Can you work these out from the model? Positions are in its coordinate system, mm. Face numbers are marked on the shaded views. A direction names the side the tool comes from. Round coordinates to 2 decimals unless told otherwise and drop trailing zeros. Loops run counter-clockwise (first coordinate to the right, second up) from the corner with the lowest first, then second, coordinate; pieces in that order, holes last.
(1) Which directions (+Z, -Z, +X, -X, +Y, -Y) give clear straight access to the entire face, cutting with the end or side of a thin tool? Please do the marked faces 5, 6 and 7.
(2) Will these pins go through, and if not, where does the flat tip stop? pin 1 Ø9 at (x, y) = (-27.5, 355) entering from +Z; pin 2 Ø14.5 at (x, y) = (-257.5, 35) entering from +Z; pin 3 Ø3 at (x, y) = (-41.5, 179) entering from -Z; pin 4 Ø21.5 at (x, y) = (-267.5, 30) entering from +Z.
(3) I want a section at B-B on x = -94.5. Write out the boundary of the cut face in (y, z), plus the area to 3 significant figures.
(4) If I drill on line 1 along Y through (x, z) = (-17, 10); line 2 along X through (y, z) = (195, 36); line 3 along X through (y, z) = (349, 14.25), over which ranges is the centre line in solid material (lowest first)?
(5) Thinking about a two-plate mould opening in Y: for the marked faces 1, 2, 3 and 4, which applies, released by +Y, released by -Y, zero draft, split by the parting line, or undercut?
(6) I want a section at A-A on y = 195. Write out the boundary of the cut face in (x, z), plus the area to 3 significant figures.
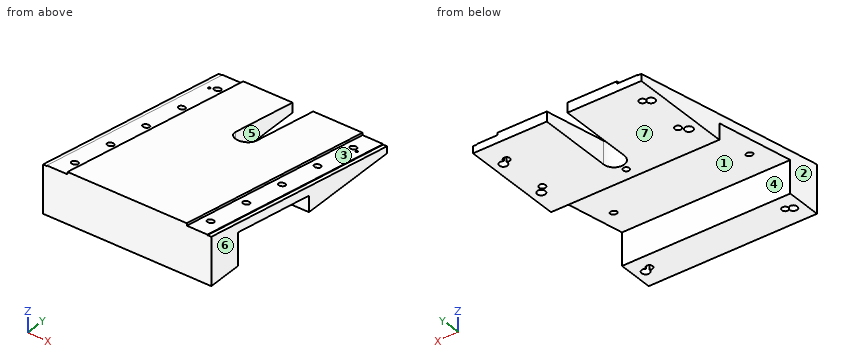
from build123d import *

# Parameters (mm, degrees)
F1_DEPTH  = 285
F3_DEPTH  = 41.5
F5_DEPTH  = 6.5
F7_DEPTH  = 41.5
F8_DEPTH  = 6.5
F13_D     = 11
F15_D     = 13.5
F15_DEPTH = 18
F15_START = 0.4782643
F15_TIP   = 4.0558091784
F17_DEPTH = 85.6227357069
F19_D     = 10
F19_DEPTH = 12
F19_TIP   = 3.0043030951


# Not quite as in the source:
# - a feature names something its author has since deleted; it is built from what else it names


with BuildPart() as f1:
    # F0 (on Right) → F1 (new body)
    with BuildSketch(Plane.YZ):
        Polygon((60, 55.2), (0, 65.8), (0, 0), (60, 0), align=None)
        Polygon((394, 17.0782642931), (0, 86.1), (0, 65.8), (60, 55.2), (219, 27.6782642931), (219, 0.4782642931), (394, 0.4782642931), align=None)
    extrude(amount=-F1_DEPTH)

    # F2 (on face) → F3 (cut)
    with BuildSketch(Plane.YZ):
        Polygon((394, 17.0782642931), (0, 86.1), (0, 82.1), (394, 13.0782642931), align=None)
    extrude(amount=-F3_DEPTH, mode=Mode.SUBTRACT)

    # F4 (on face) → F5 (cut)
    with BuildSketch(Plane.YZ):
        Polygon((394, 13.0782642931), (0, 82.1), (0, 81.1), (394, 12.0782642931), align=None)
    extrude(amount=-F5_DEPTH, mode=Mode.SUBTRACT)

    # F6 (on face) → F7 (cut)
    with BuildSketch(Plane(origin=(-285, 0, 0), x_dir=(0, -1, 0), z_dir=(-1, 0, 0))):
        Polygon((0, 86.1), (-394, 17.0782642931), (-394, 13.0782642931), (0, 82.1), align=None)
    extrude(amount=-F7_DEPTH, mode=Mode.SUBTRACT)

    # F6 (on face) → F8 (cut)
    with BuildSketch(Plane(origin=(-285, 0, 0), x_dir=(0, -1, 0), z_dir=(-1, 0, 0))):
        Polygon((0, 82.1), (-394, 13.0782642931), (-394, 12.0782642931), (0, 81.1), align=None)
    extrude(amount=-F8_DEPTH, mode=Mode.SUBTRACT)

    # F13 (through all)
    with Locations(Plane.XY.offset(86.1)):
        with Locations((-257.5, 355), (-257.5, 275), (-257.5, 195), (-27.5, 355), (-27.5, 275), (-27.5, 195), (-27.5, 115), (-27.5, 35), (-257.5, 115), (-257.5, 35)):
            Hole(F13_D / 2)

    # F15
    # its depths count from where the whole tool has entered the part; down to there all is cleared
    with Locations(Plane(origin=(0, 0, 0), x_dir=(1, 0, 0), z_dir=(0, 0, -1))):
        with Locations((-17.5, -349, 0), (-17.5, -264, -F15_START), (-17.5, -30, 0), (-267.5, -30, 0), (-267.5, -264, -F15_START), (-267.5, -349, 0)):
            Hole(F15_D / 2, depth=F15_DEPTH)
            with Locations((0, 0, -(F15_DEPTH + F15_TIP / 2))):  # 118° drill point
                Cone(0, F15_D / 2, F15_TIP, mode=Mode.SUBTRACT)

    # F16 (on face) → F17 (cut, through all)
    with BuildSketch(Plane(origin=(0, 0, 0.4782642931), x_dir=(1, 0, 0), z_dir=(0, 0, -1))):
        with BuildLine():
            Line((-160, -394), (-125, -394))
            Line((-125, -394), (-125, -266.5))
            ThreePointArc((-125, -266.5), (-142.5, -249), (-160, -266.5))
            Line((-160, -266.5), (-160, -394))
        make_face()
    extrude(amount=-F17_DEPTH, mode=Mode.SUBTRACT)

    # F19
    with Locations(Plane(origin=(0, 0, 0.4782642931), x_dir=(1, 0, 0), z_dir=(0, 0, -1))):
        with Locations((-142.5, -239)):
            Hole(F19_D / 2, depth=F19_DEPTH)
            with Locations((0, 0, -(F19_DEPTH + F19_TIP / 2))):  # 118° drill point
                Cone(0, F19_D / 2, F19_TIP, mode=Mode.SUBTRACT)


solid = f1.part
Filled sheet:
1. face 5: +Z, -Z, +Y
1. face 6: +Z, -Z, +X, +Y, -Y
1. face 7: -Z, +X, -X, +Y
2. pin 1: passes through
2. pin 2: stops at z = 77.24
2. pin 3: stops at z = 34.34
2. pin 4: stops at z = 78.73
3. outline: (0, 0) - (60, 0) - (60, 55.2) - (219, 27.68) - (219, 0.48) - (394, 0.48) - (394, 17.08) - (0, 86.1) - close
3. area: 13,700 mm2
4. line 1: y = 0 to 23.27, 36.73 to 60, 219 to 257.27, 270.73 to 342.27, 355.73 to 394
4. line 2: x = -285 to -263, -252 to -33, -22 to 0
4. line 3: x = -285 to -274.25, -260.75 to -160, -125 to -24.25, -10.75 to 0
5. face 1: undercut
5. face 2: zero draft
5. face 3: released by +Y
5. face 4: undercut
6. outline: (-285, 31.83) - (-263, 31.83) - (-263, 47.94) - (-278.5, 47.94) - (-278.5, 46.94) - (-285, 46.94) - close; (-252, 31.83) - (-33, 31.83) - (-33, 47.94) - (-41.5, 47.94) - (-41.5, 51.94) - (-243.5, 51.94) - (-243.5, 47.94) - (-252, 47.94) - close; (-22, 31.83) - (0, 31.83) - (0, 46.94) - (-6.5, 46.94) - (-6.5, 47.94) - (-22, 47.94) - close
6. area: 5,030 mm2
